Read the model definition and answer for the solid it produces. Units are mm, in the model's axes. Give positions to 0.01 mm unless a question says otherwise; leave off trailing zeros. Loops run counter-clockwise (first coordinate to the right, second up) from the corner with the lowest first, then second, coordinate; pieces in that order, holes last. Notation, with made-up numbers: (-36, 4.5) -> (18, 4.5) arc R35 ccw to (18, 39.5) -> close; hole circle Ø5 at (-3.75, -25.5). An arc over 180 degrees is marked (long way). Write each question's results on one line, items separated by ' | '. Start each with the question number.
Item 1: Section C-C on x = 38.5 is taken. Write down the section's boundary in (y, z).
Item 2: Section A-A on z = 7.25 is taken. Write down the section's boundary in (x, y).
Item 3: This flat-tipped pin is pushed along its axis until it touches: P1, Ø5, axis at x = 38, y = 1, coming from the +Z side. Where does it stop, or does it pass through?
Item 4: Section B-B on y = 11 is taken. Write down the section's boundary in (x, z).
Item 5: Find the intervals of material crossed by line 1 (Z direction, x = -50.5, y = -36); line 2 (Y direction, x = 50.5, z = 6.75), in increasing order.
```python
from build123d import *

# Parameters (mm, degrees)
F1_R     = 1.45
F2_DEPTH = 2
F3_DEPTH = 10


with BuildPart() as f2:
    # F1 (on Top) → F2 (new body)
    with BuildSketch(Plane.XY):
        with BuildLine():
            ThreePointArc((-53.202599287, 59.0909458041), (-55.9603157337, 57.9486622507), (-57.102599287, 55.1909458041))
            Line((-57.102599287, 55.1909458041), (-57.102599287, -49.8090541959))
            ThreePointArc((-57.102599287, -49.8090541959), (-55.9603157337, -52.5667706425), (-53.202599287, -53.7090541959))
            Line((-53.202599287, -53.7090541959), (51.797400713, -53.7090541959))
            ThreePointArc((51.797400713, -53.7090541959), (54.5551171596, -52.5667706425), (55.697400713, -49.8090541959))
            Line((55.697400713, -49.8090541959), (55.697400713, 55.1909458041))
            ThreePointArc((55.697400713, 55.1909458041), (54.5551171596, 57.9486622507), (51.797400713, 59.0909458041))
            Line((51.797400713, 59.0909458041), (-53.202599287, 59.0909458041))
        make_face()
        with Locations((-53.202599287, -49.8090541959)):
            Circle(F1_R, mode=Mode.SUBTRACT)
        with Locations((51.797400713, -49.8090541959)):
            Circle(F1_R, mode=Mode.SUBTRACT)
        with Locations((-53.202599287, 55.1909458041)):
            Circle(F1_R, mode=Mode.SUBTRACT)
        with Locations((51.797400713, 55.1909458041)):
            Circle(F1_R, mode=Mode.SUBTRACT)
    extrude(amount=F2_DEPTH)

    # F1 (on Top) → F3 (join)
    with BuildSketch(Plane.XY):
        with Locations((-53.202599287, 55.1909458041)):
            Circle(F1_R)
        with Locations((51.797400713, 55.1909458041)):
            Circle(F1_R)
        with Locations((-53.202599287, -49.8090541959)):
            Circle(F1_R)
        with Locations((51.797400713, -49.8090541959)):
            Circle(F1_R)
    extrude(amount=F3_DEPTH)


solid = f2.part
```
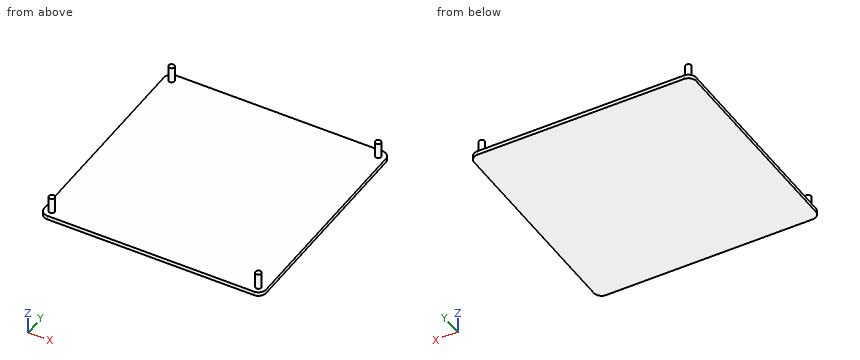
Findings:
1) outline: (-53.71, 0) -> (59.09, 0) -> (59.09, 2) -> (-53.71, 2) -> close
2) outline: circle Ø2.9 at (-53.2, -49.81); circle Ø2.9 at (-53.2, 55.19); circle Ø2.9 at (51.8, -49.81); circle Ø2.9 at (51.8, 55.19)
3) P1: z = 2
4) outline: (-57.1, 0) -> (55.7, 0) -> (55.7, 2) -> (-57.1, 2) -> close
5) line 1: 0 to 2 | line 2: -50.46 to -49.16, 54.54 to 55.84
